Part model, mm, in its own coordinate system. A direction names the side the tool comes from. Round coordinates to 2 decimals unless told otherwise and drop trailing zeros. Write each loop counter-clockwise with the first axis right and the second up, starting at its lowest first coordinate (ties: lowest second). Pieces come first, ordered by that corner, then holes.
```python
from build123d import *

# Parameters (mm, degrees)
SKETCH1_W           = 34.925
SKETCH1_H           = 12.7
BOSS_EXTRUDE1_DEPTH = 76.2
SKETCH2_W           = 28.575
SKETCH2_H           = 6.35
CUT_EXTRUDE1_DEPTH  = 74.93
FILLET1_R           = 3.175


with BuildPart() as part:
    # Sketch1 → Boss-Extrude1 (new body)
    with BuildSketch(Plane.XY):
        Rectangle(SKETCH1_W, SKETCH1_H)
    extrude(amount=BOSS_EXTRUDE1_DEPTH)

    # Sketch2 → Cut-Extrude1 (cut)
    with BuildSketch(Plane.XY.offset(76.2)):
        Rectangle(SKETCH2_W, SKETCH2_H)
    extrude(amount=-CUT_EXTRUDE1_DEPTH, mode=Mode.SUBTRACT)

    # Fillet1
    fillet1_edges = [part.edges().sort_by_distance(p)[0] for p in [
        (-17.4625, 6.35, 38.1),
        (17.4625, 6.35, 38.1),
        (0, 6.35, 76.2),
    ]]
    fillet(fillet1_edges, radius=FILLET1_R - 0.0001)  # a hair under: the kernel refuses the full size


solid = part.part
```
Q1. Cut at D-D on y = 5.25. Write the cut outline in (x, z).
Values follow:
outline: (-16.69, 0) - (16.69, 0) - (16.69, 75.43) - (-16.69, 75.43) - close
Q2. Wall check: L1, parallel to Y at x = 13, z = 10 (3 decimals); L2, parallel to X at y = -2, z = 31; L3, parallel to Z at x = -5, y = 3.5. Give the ranges that are in metal, low to high.
Values follow:
L1: y = -6.35 to -3.175, 3.175 to 6.35
L2: x = -17.46 to -14.29, 14.29 to 17.46
L3: z = 0 to 76.18
Q3. Drop flat-ended pins along their axis: pin 1 (1 mm diameter, centred on x = -0.5, y = 2, fed in from +Z); pin 2 (3 mm diameter, centred on x = 8.5, y = 5, fed in from +Z). Give the stop position or say it passes through.
Values follow:
pin 1: stops at z = 1.27
pin 2: stops at z = 76.18
Q4. Mould opens along Y. For faces 1 (the cylindrical face through (-16.557, 5.395, 38.633)), 2 (the flat face through (0, -4, 76.2)), 3 (the flat face through (0, -6.35, 38)), 4 (the flat face through (14.288, 0, 39)) say: +Y half, -Y half, draft (parallel to the pull), parting line (faces both ways), or undercut.
Values follow:
face 1: +Y half
face 2: draft
face 3: -Y half
face 4: undercut
Q5. Cut at C-C on y = 0. Write the cut outline in (x, z).
Values follow:
outline: (-17.46, 0) - (17.46, 0) - (17.46, 76.2) - (14.29, 76.2) - (14.29, 1.27) - (-14.29, 1.27) - (-14.29, 76.2) - (-17.46, 76.2) - close
Q6. Which spindle directions (+Z, -Z, +X, -X, +Y, -Y) get a long thin tool onto all of the face, cutting with end or side? Do faces 5 (the flat face through (-14.288, 0, 39)), 6 (the flat face through (-17.462, -2, 38)). Say none if no direction does.
Values follow:
face 5: +Z
face 6: +Z, -Z, -X, +Y, -Y
